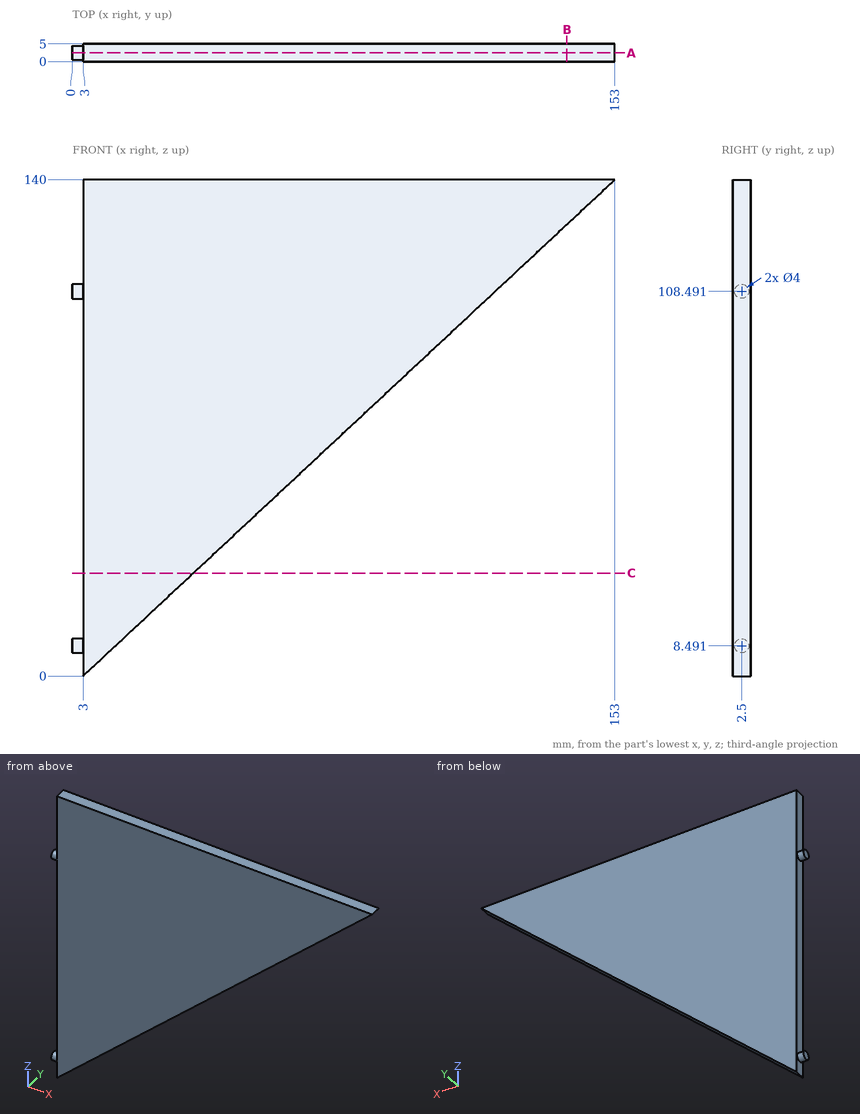
Job drawing, mm, ordinate dimensions from the low corner. One solid piece. Coordinates: 2 decimals unless noted, no trailing zeros. Write each loop counter-clockwise with the first axis right and the second up, starting at its lowest first coordinate (ties: lowest second). Pieces come first, ordered by that corner, then holes. Notation, with made-up numbers: (-21, -9.5) - (30, -9.5) arc R20 ccw to (30, 17.5) - close; hole circle Ø2 at (45, 9). An arc over 180 degrees is marked (long way). Use a Markdown table: item, result. Add a question column.
Item 1: Band-saw the part on C-C, the plane z = 29. Give the cut face in (x, y), and give its area (3 significant figures).
Item 2: Band-saw the part on B-B, the plane x = 139.5. Give the cut face in (y, z).
Item 3: Band-saw the part on A-A, the plane y = 2.5. Give the cut face in (x, z), and give its area (3 significant figures).
Item 4: Flat gauge pins, fed straight in: pin 1 (2 mm diameter, centred on y = 2, z = 61, fed in from +X); pin 2 (3 mm diameter, centred on x = 33, y = 3, fed in from -Z). Where does each tip first touch, or does it go through?
Item 5: Drill centre lines: L1, parallel to X at y = 2.25, z = 123 (1 decimal); L2, parallel to X at y = 3.7, z = 72.5; L3, parallel to Z at x = 129, y = 2.1. Where is each one in solid material? Low to high. Write a range as from..to.
Numbers:
| question | item | result |
|---|---|---|
| 1 | outline | (3, 0) - (34.07, 0) - (34.07, 5) - (3, 5) - close |
| 1 | area | 155 mm2 |
| 2 | outline | (0, 127.4) - (5, 127.4) - (5, 140) - (0, 140) - close |
| 3 | outline | (0, 6.49) - (3, 6.49) - (3, 0) - (153, 140) - (3, 140) - (3, 110.49) - (0, 110.49) - (0, 106.49) - (3, 106.49) - (3, 10.49) - (0, 10.49) - close |
| 3 | area | 10,500 mm2 |
| 4 | pin 1 | x = 69.43 |
| 4 | pin 2 | z = 26.6 |
| 5 | L1 | 3..134.8 |
| 5 | L2 | 3..80.68 |
| 5 | L3 | 117.6..140 |
